```python
from build123d import *

# Parameters (mm, degrees)
F1_DEPTH = 76.2
F3_D     = 6.35
F3_DEPTH = 19.05
F3_TIP   = 1.9077324654
F5_DEPTH = 3.175
F7_DEPTH = 3.175
F9_D     = 6.35
F9_DEPTH = 19.05
F9_TIP   = 1.9077324654


with BuildPart() as f1:
    # F0 (on Front) → F1 (new body)
    with BuildSketch(Plane.XZ):
        Polygon((1.6724448999, 115.5307332167), (0, 0), (38.1, 0), (38.1, 133.35), (20.0152, 133.35), align=None)
    extrude(amount=F1_DEPTH)

    # F3
    with Locations(Plane(origin=(-56.9291441584, 0, 58.6015890583), x_dir=(0.7172678422, 0, 0.6967975621), z_dir=(-0.6967975621, 0, 0.7172678422))):
        with Locations((94.487669207, -6.35), (94.487669207, -69.85)):
            Hole(F3_D / 2, depth=F3_DEPTH)
            with Locations((0, 0, -(F3_DEPTH + F3_TIP / 2))):  # 118° drill point
                Cone(0, F3_D / 2, F3_TIP, mode=Mode.SUBTRACT)

    # F4 (on face) → F5 (join)
    with BuildSketch(Plane.XZ.offset(76.2)):
        Polygon((20.0152, 133.35), (1.6724448999, 115.5307332167), (0, 0), (38.1, 0), (38.1, 133.35), align=None)
    extrude(amount=F5_DEPTH)

    # F6 (on face) → F7 (join)
    with BuildSketch(Plane(origin=(0, 0, 0), x_dir=(-1, 0, 0), z_dir=(0, 1, 0))):
        Polygon((-38.1, 0), (0, 0), (-1.6724448999, 115.5307332167), (-20.0152, 133.35), (-38.1, 133.35), align=None)
    extrude(amount=F7_DEPTH)

    # F9
    with Locations(Plane(origin=(0, 0, 0), x_dir=(1, 0, 0), z_dir=(0, 0, -1))):
        with Locations((19.05, 9.525), (19.05, 66.675)):
            Hole(F9_D / 2, depth=F9_DEPTH)
            with Locations((0, 0, -(F9_DEPTH + F9_TIP / 2))):  # 118° drill point
                Cone(0, F9_D / 2, F9_TIP, mode=Mode.SUBTRACT)


solid = f1.part
```
Verification items for the finished model (mm, model axes). A direction names the side the tool comes from. Coordinates: 2 decimals unless noted, no trailing zeros. Loops run counter-clockwise (first coordinate to the right, second up) from the corner with the lowest first, then second, coordinate; pieces in that order, holes last. Notation, with made-up numbers: (62, 40.25) -> (101, 40.25) arc R26 cw to (101, 79.25) -> close; hole circle Ø8 at (79, 83.25). An arc over 180 degrees is marked (long way). Answer in a Markdown table with one row per item. Add a question column.
1. Section check C-C, the plane z = 107. Enter the section's corners in (x, y) (3 decimals).
2. Section check B-B, the plane y = -47. Enter the section's corners in (x, z).
3. Access from +Z, -Z, +X, -X, +Y, -Y to the whole of each face (thin tool, end or side, straight path). Record for faces 4 (the face through (24.92, -5.98, 109.36)), 5 (the face through (16.02, -10.48, 9.66)), 6 (the face through (19, -39, 0)).
4. Material ranges on probe 1 along Y at (x, z) = (19.05, 12) (3 decimals); probe 2 along X at (y, z) = (-65.5, 13); probe 3 along X at (y, z) = (-32.5, 74), recorded low to high. Write a range as [from, to].
5. Section check A-A, the plane z = 14. Enter the section's corners in (x, y) (3 decimals).
6. Depth check by flat-ended pin: P1, Ø6, axis at y = -64.5, z = 37, coming from the -X side; P2, Ø1, axis at y = -49, z = 85, coming from the -X side; P3, Ø10, axis at x = 11.5, y = -64.5, coming from the +Z side. Enter the tip coordinate at first touch or a pass-through.
7. Draft check along Z on faces 1 (the face through (19, -79.375, 68)), 2 (the face through (18.9, -66.1, 20.6)), 3 (the face through (24.82, -69.83, 109.26)). Enter one of: +Z half, -Z half, draft (parallel to the pull), parting line (faces both ways), or undercut.
8. Section check D-D, the plane z = 58.5. Enter the section's corners in (x, y) (3 decimals).
Derived:
| question | item | result |
|---|---|---|
| 1 | outline | (1.549, -79.375) -> (38.1, -79.375) -> (38.1, 3.175) -> (1.549, 3.175) -> close |
| 2 | outline | (0, 0) -> (38.1, 0) -> (38.1, 133.35) -> (20.02, 133.35) -> (1.67, 115.53) -> close |
| 3 | face 4 | none |
| 3 | face 5 | -Z |
| 3 | face 6 | -Z, +X, -X, +Y, -Y |
| 4 | probe 1 | y = [-79.375, -69.85], [-63.5, -12.7], [-6.35, 3.175] |
| 4 | probe 2 | x = [0.19, 16.1], [22, 38.1] |
| 4 | probe 3 | x = [1.07, 38.1] |
| 5 | outline | (0.203, -79.375) -> (38.1, -79.375) -> (38.1, 3.175) -> (0.203, 3.175) -> close; hole circle Ø6.35 at (19.05, -66.675); hole circle Ø6.35 at (19.05, -9.525) |
| 6 | P1 | stops at x = 0.49 |
| 6 | P2 | stops at x = 1.22 |
| 6 | P3 | stops at z = 129.94 |
| 7 | face 1 | draft |
| 7 | face 2 | -Z half |
| 7 | face 3 | undercut |
| 8 | outline | (0.847, -79.375) -> (38.1, -79.375) -> (38.1, 3.175) -> (0.847, 3.175) -> close |
